Here's how the part is built. I have some questions about the finished solid (model axes, mm). A direction names the side the tool comes from. Coordinates: 2 decimals unless noted, no trailing zeros. Write each loop counter-clockwise with the first axis right and the second up, starting at its lowest first coordinate (ties: lowest second). Pieces come first, ordered by that corner, then holes. Notation, with made-up numbers: (-28.75, 21.25) -> (-5.75, 21.25) arc R4 ccw to (-5.75, 28.25) -> close; hole circle Ø2 at (25.5, -23). An arc over 180 degrees is marked (long way). Put each result on its own line as item: value. Start each with the question number.
Item 1: I want a section at A-A, the plane z = 0. List the corners of the cut face in (x, y) for me, then the cut area to 3 significant figures.
Item 2: On a 3-axis mill with a long thin cutter (end or side, diameter ignored), from which of +Z, -Z, +X, -X, +Y, -Y can I reach the whole of each face in a straight line? I mean faces 4 (the face through (-148, -25, 0)), 5 (the face through (-12, -20, -145)), 6 (the face through (-108.49, -10.14, -107.68)). Say none if no direction works.
Item 3: I need wall thicknesses on line 1 (Z direction, x = -105, y = -12.25); line 2 (Z direction, x = -148.65, y = -25); line 3 (Z direction, x = -137.25, y = -25). Which ranges of each line are inside material? Lowest first, please. Write a range as [from, to].
Item 4: For pin 1 (3 mm diameter, centred on y = -20.5, z = 70.5, fed in from +X); pin 2 (10 mm diameter, centred on x = 143.5, y = -34.5, fed in from -Z); pin 3 (4 mm diameter, centred on x = -105, z = 105, fed in from -Y); pin 4 (1.5 mm diameter, centred on x = 64.5, y = -26, fed in from -Z), each with a flat end and sliding along its axis, tell me the tip position at first contact or that it passes through.
Item 5: I want a section at B-B, the plane x = 69. List the corners of the cut face in (y, z) for me.
Item 6: If we mould it in two halves opening along Y, with no side actions, what happens to faces 1 (the face through (-134.297, -25.716, -74.547)), 2 (the face through (-149.01, -30.08, -2.11)), 3 (the face through (-12, -40, -150))? For each: released by +Y, released by -Y, zero draft, split by the parting line, or undercut.
Item 7: I want a section at C-C, the plane z = 105. State how many separate pieces and enclosed holes the cut face has, then the cut area to 3 significant figures.
from build123d import *

# Parameters (mm, degrees)
F0_W      = 300
F0_H      = 300
F1_DEPTH  = 50
F3_DEPTH  = 50
F4_R      = 5.5
F5_DEPTH  = 2
F7_D      = 11
F7_DEPTH  = 30
F7_TIP    = 3.3047334047
F8_W      = 41
F8_H      = 220
F9_DEPTH  = 20
F10_R     = 3.5
F11_DEPTH = 50
F12_R     = 20
F13_W     = 280
F13_H     = 10
F14_DEPTH = 10
F16_D     = 8.8
F16_DEPTH = 20
F16_TIP   = 2.6437867237
F18_D     = 8.8
F18_DEPTH = 20
F18_TIP   = 2.6437867237
F19_R     = 7
F20_DEPTH = 1


with BuildPart() as f1:
    # F0 (on Front) → F1 (new body)
    with BuildSketch(Plane.XZ):
        Rectangle(F0_W, F0_H)
    extrude(amount=F1_DEPTH)

    # F2 (on face) → F3 (cut)
    with BuildSketch(Plane.XZ.offset(50)):
        with BuildLine():
            ThreePointArc((55.8586385441, 32.25), (69.609943325, 20.8997497965), (87.4351784027, 21.3328286376))
            ThreePointArc((87.4351784027, 21.3328286376), (83.5311930437, 33.5043249252), (77.9422863406, 45))
            Line((77.9422863406, 45), (55.8586385441, 32.25))
        make_face()
        with BuildLine():
            ThreePointArc((77.9422863406, 45), (83.5311930437, 33.5043249252), (87.4351784027, 21.3328286376))
            ThreePointArc((87.4351784027, 21.3328286376), (99.0647713694, 30.7139709433), (103.4422863406, 45))
            ThreePointArc((103.4422863406, 45), (102.573394911, 51.5998856501), (100.0259341371, 57.75))
            Line((100.0259341371, 57.75), (77.9422863406, 45))
        make_face()
        with BuildLine():
            Line((55.8586385441, 32.25), (77.9422863406, 45))
            ThreePointArc((77.9422863406, 45), (70.7811930437, 55.5879727217), (62.1923607361, 65.0546713624))
            ThreePointArc((62.1923607361, 65.0546713624), (52.904685919, 49.8341043772), (55.8586385441, 32.25))
        make_face()
        with BuildLine():
            ThreePointArc((62.1923607361, 65.0546713624), (70.7811930437, 55.5879727217), (77.9422863406, 45))
            Line((77.9422863406, 45), (100.0259341371, 57.75))
            ThreePointArc((100.0259341371, 57.75), (82.7763907178, 70.0376004216), (62.1923607361, 65.0546713624))
        make_face()
        with BuildLine():
            ThreePointArc((0, 90), (12.75, 89.0922976469), (25.2428176666, 86.3875))
            ThreePointArc((25.2428176666, 86.3875), (25.4356231543, 88.1891784321), (25.5, 90))
            ThreePointArc((25.5, 90), (-1.8108215679, 115.4356231543), (-25.2428176666, 86.3875))
            ThreePointArc((-25.2428176666, 86.3875), (-12.75, 89.0922976469), (0, 90))
        make_face()
        with BuildLine():
            ThreePointArc((0, 64.5), (16.705257406, 70.7338541737), (25.2428176666, 86.3875))
            ThreePointArc((25.2428176666, 86.3875), (12.75, 89.0922976469), (0, 90))
            Line((0, 90), (0, 64.5))
        make_face()
        with BuildLine():
            ThreePointArc((-25.2428176666, 86.3875), (-16.705257406, 70.7338541737), (0, 64.5))
            Line((0, 64.5), (0, 90))
            ThreePointArc((0, 90), (-12.75, 89.0922976469), (-25.2428176666, 86.3875))
        make_face()
        with BuildLine():
            Line((-77.9422863406, 45), (-55.8586385441, 32.25))
            ThreePointArc((-55.8586385441, 32.25), (-53.3111777702, 38.4001143499), (-52.4422863406, 45))
            ThreePointArc((-52.4422863406, 45), (-55.0089797439, 56.1495940977), (-62.1923607361, 65.0546713624))
            ThreePointArc((-62.1923607361, 65.0546713624), (-70.7811930437, 55.5879727217), (-77.9422863406, 45))
        make_face()
        with BuildLine():
            Line((-100.0259341371, 57.75), (-77.9422863406, 45))
            ThreePointArc((-77.9422863406, 45), (-70.7811930437, 55.5879727217), (-62.1923607361, 65.0546713624))
            ThreePointArc((-62.1923607361, 65.0546713624), (-82.7763907178, 70.0376004216), (-100.0259341371, 57.75))
        make_face()
        with BuildLine():
            ThreePointArc((-87.4351784027, 21.3328286376), (-69.609943325, 20.8997497965), (-55.8586385441, 32.25))
            Line((-55.8586385441, 32.25), (-77.9422863406, 45))
            ThreePointArc((-77.9422863406, 45), (-83.5311930437, 33.5043249252), (-87.4351784027, 21.3328286376))
        make_face()
        with BuildLine():
            ThreePointArc((-87.4351784027, 21.3328286376), (-83.5311930437, 33.5043249252), (-77.9422863406, 45))
            Line((-77.9422863406, 45), (-100.0259341371, 57.75))
            ThreePointArc((-100.0259341371, 57.75), (-102.0425365441, 36.6676569844), (-87.4351784027, 21.3328286376))
        make_face()
        with BuildLine():
            ThreePointArc((-62.1923607361, -65.0546713624), (-70.7811930437, -55.5879727217), (-77.9422863406, -45))
            ThreePointArc((-77.9422863406, -45), (-83.5311930437, -33.5043249252), (-87.4351784027, -21.3328286376))
            ThreePointArc((-87.4351784027, -21.3328286376), (-100.0259341371, -57.75), (-62.1923607361, -65.0546713624))
        make_face()
        with BuildLine():
            Line((-77.9422863406, -45), (-55.8586385441, -32.25))
            ThreePointArc((-55.8586385441, -32.25), (-69.609943325, -20.8997497965), (-87.4351784027, -21.3328286376))
            ThreePointArc((-87.4351784027, -21.3328286376), (-83.5311930437, -33.5043249252), (-77.9422863406, -45))
        make_face()
        with BuildLine():
            ThreePointArc((-52.4422863406, -45), (-53.3111777702, -38.4001143499), (-55.8586385441, -32.25))
            Line((-55.8586385441, -32.25), (-77.9422863406, -45))
            ThreePointArc((-77.9422863406, -45), (-70.7811930437, -55.5879727217), (-62.1923607361, -65.0546713624))
            ThreePointArc((-62.1923607361, -65.0546713624), (-55.0089797439, -56.1495940977), (-52.4422863406, -45))
        make_face()
        with BuildLine():
            ThreePointArc((25.5, -90), (25.4356231543, -88.1891784321), (25.2428176666, -86.3875))
            ThreePointArc((25.2428176666, -86.3875), (12.75, -89.0922976469), (0, -90))
            ThreePointArc((0, -90), (-12.75, -89.0922976469), (-25.2428176666, -86.3875))
            ThreePointArc((-25.2428176666, -86.3875), (-1.8108215679, -115.4356231543), (25.5, -90))
        make_face()
        with BuildLine():
            Line((0, -90), (0, -64.5))
            ThreePointArc((0, -64.5), (-16.705257406, -70.7338541737), (-25.2428176666, -86.3875))
            ThreePointArc((-25.2428176666, -86.3875), (-12.75, -89.0922976469), (0, -90))
        make_face()
        with BuildLine():
            ThreePointArc((25.2428176666, -86.3875), (16.705257406, -70.7338541737), (0, -64.5))
            Line((0, -64.5), (0, -90))
            ThreePointArc((0, -90), (12.75, -89.0922976469), (25.2428176666, -86.3875))
        make_face()
        with BuildLine():
            ThreePointArc((103.4422863406, -45), (99.0647713694, -30.7139709433), (87.4351784027, -21.3328286376))
            ThreePointArc((87.4351784027, -21.3328286376), (83.5311930437, -33.5043249252), (77.9422863406, -45))
            ThreePointArc((77.9422863406, -45), (70.7811930437, -55.5879727217), (62.1923607361, -65.0546713624))
            ThreePointArc((62.1923607361, -65.0546713624), (89.0918804383, -67.9333065967), (103.4422863406, -45))
        make_face()
        with BuildLine():
            ThreePointArc((62.1923607361, -65.0546713624), (70.7811930437, -55.5879727217), (77.9422863406, -45))
            Line((77.9422863406, -45), (55.8586385441, -32.25))
            ThreePointArc((55.8586385441, -32.25), (52.904685919, -49.8341043772), (62.1923607361, -65.0546713624))
        make_face()
        with BuildLine():
            ThreePointArc((77.9422863406, -45), (83.5311930437, -33.5043249252), (87.4351784027, -21.3328286376))
            ThreePointArc((87.4351784027, -21.3328286376), (69.609943325, -20.8997497965), (55.8586385441, -32.25))
            Line((55.8586385441, -32.25), (77.9422863406, -45))
        make_face()
    extrude(amount=-F3_DEPTH, mode=Mode.SUBTRACT)

    # F4 (on face) → F5 (cut)
    with BuildSketch(Plane(origin=(-150, 0, 0), x_dir=(0, -1, 0), z_dir=(-1, 0, 0))):
        with Locations((25, 0)):
            Circle(F4_R)
    extrude(amount=-F5_DEPTH, mode=Mode.SUBTRACT)

    # F7
    with Locations(Plane(origin=(-150, 0, 0), x_dir=(0, -1, 0), z_dir=(-1, 0, 0))):
        with Locations((25, 80), (25, -80)):
            Hole(F7_D / 2, depth=F7_DEPTH)
            with Locations((0, 0, -(F7_DEPTH + F7_TIP / 2))):  # 118° drill point
                Cone(0, F7_D / 2, F7_TIP, mode=Mode.SUBTRACT)

    # F8 (on face) → F9 (cut)
    with BuildSketch(Plane.YZ.offset(150)):
        with Locations((-25, 0)):
            Rectangle(F8_W, F8_H)
    extrude(amount=-F9_DEPTH, mode=Mode.SUBTRACT)

    # F10 (on face) → F11 (cut)
    with BuildSketch(Plane.XZ.offset(50)):
        with Locations((-105, 105)):
            Circle(F10_R)
        with Locations((105, 105)):
            Circle(F10_R)
        with Locations((-105, -105)):
            Circle(F10_R)
        with Locations((105, -105)):
            Circle(F10_R)
        Circle(F10_R)
    extrude(amount=-F11_DEPTH, mode=Mode.SUBTRACT)

    # F12
    f12_edges = [f1.edges().sort_by_distance(p)[0] for p in [
        (150, -25, 150),
        (150, -25, -150),
    ]]
    fillet(f12_edges, radius=F12_R)

    # F13 (on face) → F14 (cut)
    with BuildSketch(Plane(origin=(0, 0, -150), x_dir=(1, 0, 0), z_dir=(0, 0, -1))):
        with Locations((-10, 25)):
            Rectangle(F13_W, F13_H)
    extrude(amount=-F14_DEPTH, mode=Mode.SUBTRACT)

    # F16
    with Locations(Plane.XZ.offset(50)):
        with Locations((-105, 105), (105, 105), (0, 0), (-105, -105), (105, -105)):
            Hole(F16_D / 2, depth=F16_DEPTH)
            with Locations((0, 0, -(F16_DEPTH + F16_TIP / 2))):  # 118° drill point
                Cone(0, F16_D / 2, F16_TIP, mode=Mode.SUBTRACT)

    # F18
    with Locations(Plane(origin=(0, 0, 0), x_dir=(-1, 0, 0), z_dir=(0, 1, 0))):
        with Locations((-105, 105), (105, 105), (0, 0), (-105, -105), (105, -105)):
            Hole(F18_D / 2, depth=F18_DEPTH)
            with Locations((0, 0, -(F18_DEPTH + F18_TIP / 2))):  # 118° drill point
                Cone(0, F18_D / 2, F18_TIP, mode=Mode.SUBTRACT)

    # F19 (on face) → F20 (cut)
    with BuildSketch(Plane(origin=(-150, 0, 0), x_dir=(0, -1, 0), z_dir=(-1, 0, 0))):
        with Locations((25, 80)):
            Circle(F19_R)
        with Locations((25, -80)):
            Circle(F19_R)
    extrude(amount=-F20_DEPTH, mode=Mode.SUBTRACT)


solid = f1.part
Calculated:
1. outline: (-150, -50) -> (-4.4, -50) -> (-4.4, -30) -> (-3.5, -29.46) -> (-3.5, -20.54) -> (-4.4, -20) -> (-4.4, 0) -> (-150, 0) -> (-150, -19.5) -> (-148, -19.5) -> (-148, -30.5) -> (-150, -30.5) -> close; (3.5, -29.46) -> (4.4, -30) -> (4.4, -50) -> (150, -50) -> (150, -45.5) -> (130, -45.5) -> (130, -4.5) -> (150, -4.5) -> (150, 0) -> (4.4, 0) -> (4.4, -20) -> (3.5, -20.54) -> close
1. area: 13,700 mm2
2. face 4: -X
2. face 5: -Z, -X
2. face 6: +Y
3. line 1: z = [-150, -109.4], [-100.6, 100.6], [109.4, 150]
3. line 2: z = [-140, -85.5], [-74.5, -5.5], [5.5, 74.5], [85.5, 150]
3. line 3: z = [-140, -85.5], [-74.5, 74.5], [85.5, 150]
4. pin 1: stops at x = 130
4. pin 2: stops at z = -148.1
4. pin 3: passes through
4. pin 4: stops at z = -140
5. outline: (-50, -150) -> (-30, -150) -> (-30, -140) -> (-20, -140) -> (-20, -150) -> (0, -150) -> (0, -68.88) -> (-50, -68.88) -> close; (-50, -21.12) -> (0, -21.12) -> (0, 21.12) -> (-50, 21.12) -> close; (-50, 68.88) -> (0, 68.88) -> (0, 150) -> (-50, 150) -> close
6. face 1: undercut
6. face 2: undercut
6. face 3: zero draft
7. separate pieces: 4
7. enclosed holes: 0
7. area: 11,300 mm2
